from build123d import *

# Parameters (mm, degrees)
F0_W     = 1219.2
F0_H     = 609.6
F1_DEPTH = 12.7
F2_D     = 152.4
F3_D     = 6.35


with BuildPart() as f1:
    # F0 (on Top) → F1 (new body)
    with BuildSketch(Plane.XY):
        Rectangle(F0_W, F0_H)
    extrude(amount=F1_DEPTH)

    # F2 (through all)
    with Locations(Plane(origin=(0, 0, 0), x_dir=(1, 0, 0), z_dir=(0, 0, -1))):
        with Locations((-381, 0)):
            Hole(F2_D / 2)

    # F3 (through all)
    with Locations(Plane(origin=(0, 0, 0), x_dir=(1, 0, 0), z_dir=(0, 0, -1))):
        with Locations((-558.8, 285.75), (-279.4, 285.75), (0, 285.75), (279.4, 285.75), (558.8, 285.75), (558.8, -285.75), (279.4, -285.75), (0, -285.75), (-279.4, -285.75), (-558.8, -285.75), (-590.55, 133.35), (-590.55, 0), (-590.55, -133.35), (590.55, 133.35), (590.55, 0), (590.55, -133.35)):
            Hole(F3_D / 2)


solid = f1.part
Design review of the part built by this model. Coordinates are the model's own, in mm. Give positions to 0.01 mm unless a question says otherwise; leave off trailing zeros. Loops run counter-clockwise (first coordinate to the right, second up) from the corner with the lowest first, then second, coordinate; pieces in that order, holes last. Notation, with made-up numbers: M 38,78.5 L 50,78.5 A35 cw 50,116.5 Z; hole C -39,16 d6. An arc over 180 degrees is marked long. One line per question, with ' | ' between items. Start each with the question number.
1. Insertion check: P1, Ø5, axis at x = 590.55, y = 133.35, coming from the +Z side. The pin has a flat end and moves straight along its axis. Give the tip position at first contact, or say it passes through.
2. Add section A-A (x = -318). Write out the cut boundary in (y, z), plus the area to 3 significant figures.
3. To check wall thickness, follow L1, parallel to Y at x = -590.55, z = 9.5 (3 decimals); L2, parallel to X at y = 133.35, z = 7.25 (3 decimals); L3, parallel to Y at x = 0, z = 5.75 (3 decimals). State the ranges of each line that lie inside material, in increasing order.
4. The part is to be moulded in two halves that separate along Y. For faces 1 (the face through (-9, 4, 12.7)), 2 (the face through (-304.874, -3.35, 6.439)), say which applies: released by +Y, released by -Y, zero draft, split by the parting line, or undercut.
5. Add section B-B (z = 6.25). Give the number of separate pieces and of enclosed holes in the cut face, plus the area to 3 significant figures.
Worked out:
1) P1: passes through
2) outline: M -304.8,0 L -42.87,0 L -42.87,12.7 L -304.8,12.7 Z; M 42.87,0 L 304.8,0 L 304.8,12.7 L 42.87,12.7 Z | area: 6,650 mm²
3) L1: y = -304.8 to -136.525, -130.175 to -3.175, 3.175 to 130.175, 136.525 to 304.8 | L2: x = -609.6 to -593.725, -587.375 to 587.375, 593.725 to 609.6 | L3: y = -304.8 to -288.925, -282.575 to 282.575, 288.925 to 304.8
4) face 1: zero draft | face 2: undercut
5) separate pieces: 1 | enclosed holes: 17 | area: 724,000 mm²
